```python
from build123d import *

# Parameters (mm, degrees)
CROQUIS1_R              = 2.5
BRIDA_BASE1_DEPTH       = 15
REDONDEO1_R             = 7.5
CHAFL_N1_SIZE           = 0.75
SALIENTE_EXTRUIR1_DEPTH = 5
REDONDEO2_R             = 1


# Sheet-metal steps are written as plain solids
with BuildPart() as part:
    # Croquis1 → Brida base1 (new body)
    with BuildSketch(Plane.XY):
        with BuildLine():
            Line((0, 30), (0, 18))
            Line((0, 18), (14, 18))
            ThreePointArc((14, 18), (17, 15), (14, 12))
            Line((14, 12), (0, 12))
            Line((0, 12), (0, 0))
            Line((0, 0), (20, 0))
            Line((20, 0), (20, 30))
            Line((20, 30), (0, 30))
        make_face()
        with Locations(Location((10, 3.25, 0), (0, 0, 180))):
            Circle(CROQUIS1_R, mode=Mode.SUBTRACT)
        with Locations((10, 26.75)):
            Circle(CROQUIS1_R, mode=Mode.SUBTRACT)
    extrude(amount=-BRIDA_BASE1_DEPTH)

    # Redondeo1
    redondeo1_edges = [part.edges().sort_by_distance(p)[0] for p in [
        (0, 30, -7.5),
        (20, 30, -7.5),
        (20, 0, -7.5),
        (0, 0, -7.5),
    ]]
    fillet(redondeo1_edges, radius=REDONDEO1_R)

    # Chaflán1
    chafl_n1_edges = [part.edges().sort_by_distance(p)[0] for p in [
        (7, 18, -15),
        (12.5, 3.25, -15),
        (12.5, 3.25, 0),
        (17, 15, -15),
        (7.5, 26.75, -15),
        (7.5, 26.75, 0),
        (7, 12, -15),
    ]]
    chamfer(chafl_n1_edges, length=CHAFL_N1_SIZE - 0.0001)  # a hair under: the kernel refuses the full size

    # Croquis2 → Saliente-Extruir1 (add)
    with BuildSketch(Plane(origin=(0, 0, 0), x_dir=(-1, 0, 0), z_dir=(0, 0, -1))):
        with BuildLine():
            Line((0, 18), (-14, 18))
            ThreePointArc((-14, 18), (-17, 15), (-14, 12))
            Line((-14, 12), (0, 12))
            Line((0, 12), (0, 18))
        make_face()
    extrude(amount=SALIENTE_EXTRUIR1_DEPTH)

    # Redondeo2
    redondeo2_edges = [part.edges().sort_by_distance(p)[0] for p in [
        (7, 18, -5),
        (17, 15, -5),
        (7, 12, -5),
    ]]
    fillet(redondeo2_edges, radius=REDONDEO2_R)


solid = part.part
```
Source: CAD feature listing. Evaluate the final solid. Frame: model axes, mm. A direction names the side the tool comes from. Give positions to 0.01 mm unless a question says otherwise; leave off trailing zeros. Order: outer loops, then holes, each group sorted by start corner. A loop starts at its lowest first (then second) coordinate and runs counter-clockwise, first axis right, second up.
(1) Material intervals for line 1 along Y through (x, z) = (10, -9.5); line 2 along Y through (x, z) = (10, -4.75); line 3 along Y through (x, z) = (8, -2), sorted ascending.
(2) Contact query for flat-ended pins moving along their axis: P1, Ø3, axis at x = 17, z = -6.5, coming from the +Y side; P2, Ø4.5, axis at x = 10, y = 3.25, coming from the -Z side; P3, Ø2, axis at x = 3, z = -13, coming from the -Y side; P4, Ø1, axis at y = 4, z = -10.5, coming from the +X side. Output: stop coordinate, or through.
(3) Section query A-A (x = 10). State how many separate pieces and enclosed holes the cut face has, plus the area to 3 significant figures.
(4) Section query D-D (y = 15). Return the cut outline in (x, z), plus the area to 3 significant figures.
(5) Pull-direction query (X, two-part tool) for faces 1 (the face through (7.098, 17.715, -5.301)), 2 (the face through (12.498, 3.14, -7.405)), 3 (the face through (17.745, 27.861, -7.605)), 4 (the face through (17.13, 15.07, -14.38)); classes: +X half, -X half, draft (parallel to the pull), parting line (faces both ways), or undercut.
(6) Section query C-C (y = 26.75). Return the cut outline in (x, z).
(7) Access query for faces 5 (the face through (9.67, 29.23, -7.41)), 6 (the face through (17, 15, -10)). Directions: +Z, -Z, +X, -X, +Y, -Y. A direction counts if a zero-diameter tool reaches every point of the face in a straight line with its end or side. Return the directions, or none.
(8) Section query B-B (z = -12). Return the cut outline in (x, y).
Outcome:
1. line 1: y = 0 to 0.75, 5.75 to 12, 18 to 24.25, 29.25 to 30
1. line 2: y = 0 to 0.75, 5.75 to 24.25, 29.25 to 30
1. line 3: y = 0 to 1.75, 4.75 to 25.25, 28.25 to 30
2. P1: stops at y = 29.37
2. P2: passes through
2. P3: stops at y = 0.87
2. P4: stops at x = 19.37
3. separate pieces: 3
3. enclosed holes: 0
3. area: 238 mm2
4. outline: (0, -5) - (16, -5) arc R1 cw to (17, -6) - (17, -14.25) - (17.75, -15) - (20, -15) - (20, 0) - (0, 0) - close
4. area: 130 mm2
5. face 1: draft
5. face 2: undercut
5. face 3: +X half
5. face 4: -X half
6. outline: (1.32, -15) - (6.75, -15) - (7.5, -14.25) - (7.5, -0.75) - (6.75, 0) - (1.32, 0) - close; (12.5, -14.25) - (13.25, -15) - (18.68, -15) - (18.68, 0) - (13.25, 0) - (12.5, -0.75) - close
7. face 5: +Z, -Z
7. face 6: -Z, -X
8. outline: (0, 7.5) arc R7.5 ccw to (7.5, 0) - (12.5, 0) arc R7.5 ccw to (20, 7.5) - (20, 22.5) arc R7.5 ccw to (12.5, 30) - (7.5, 30) arc R7.5 ccw to (0, 22.5) - (0, 18) - (14, 18) arc R3 cw to (14, 12) - (0, 12) - close; hole circle Ø5 at (10, 3.25); hole circle Ø5 at (10, 26.75)
